Source: CAD feature listing. Evaluate the final solid. Frame: model axes, mm. A direction names the side the tool comes from. Round coordinates to 2 decimals unless told otherwise and drop trailing zeros. Order: outer loops, then holes, each group sorted by start corner. A loop starts at its lowest first (then second) coordinate and runs counter-clockwise, first axis right, second up. Notation, with made-up numbers: M 47,16.5 L 87,16.5 A22 ccw 87,39.5 Z; hole C -15,80 d9. An arc over 180 degrees is marked long. Use one line per item in the form item = value. Start each with the question number.
Q1. Section C-C (x = 38.5). Return the cut outline in (y, z), plus the area to 3 significant figures.
Q2. Material intervals for probe 1 along Y at (x, z) = (53.5, 0); probe 2 along X at (y, z) = (34, 315); probe 3 along X at (y, z) = (-11, 305.5), sorted ascending.
Q3. Section D-D (y = 18.5). Return the cut outline in (x, z).
Q4. Contact query for flat-ended pins moving along their axis: pin 1 (18 mm diameter, centred on y = 3.5, z = 301, fed in from +X); pin 2 (3.5 mm diameter, centred on y = -1, z = -1.5, fed in from -X); pin 3 (12 mm diameter, centred on x = 21, z = 171.5, fed in from +Y). Output: stop coordinate, or through.
Q5. Pull-direction query (Z, two-part tool) for faces 6 (the flat face through (30, -30, 157)), 7 (the cylindrical face through (-4.93, -3.651, 305.217)), 8 (the flat face through (0, -8, 311)); classes: pulls with the +Z half, pulls with the -Z half, needs draft (parallel to the pull), parting line crosses it, or undercut.
Q6. Section B-B (y = 0). Return the cut outline in (x, z).
Q7. Reachability of faces 1 (the flat face through (60, 30, -6)), 2 (the cylindrical face through (5, 0, -6)), 3 (the flat face through (50, 0, 0)), 4 (the flat face through (0, 1, -8)), 5 (the flat face through (30, 30, 157)) from +Z, -Z, +X, -X, +Y, -Y: full face, straight path, thin tool, end or side. Return the list, or none.
Q8. Section A-A (z = 0). Return the cut outline in (x, y).
from build123d import *

# Parameters (mm, degrees)
SKETCH1_R             = 40
BOSS_EXTRUDE1_DEPTH   = 60
BOSS_EXTRUDE1_2_DEPTH = 60
BOSS_EXTRUDE2_START   = -121.840385
SKETCH5_W             = 40
SKETCH5_H             = 60
BOSS_EXTRUDE2_DEPTH   = 257.063378
SKETCH7_R             = 6
CUT_EXTRUDE5_DEPTH    = 10
SKETCH8_R             = 6
BOSS_EXTRUDE3_DEPTH   = 10
SKETCH2_R             = 30
CUT_EXTRUDE6_DEPTH    = 10


with BuildPart() as part:
    # Sketch1 → Boss-Extrude1 (new body)
    with BuildSketch(Plane(origin=(0, 0, 0), x_dir=(0, 0, -1), z_dir=(1, 0, 0))):
        Circle(SKETCH1_R)
    extrude(amount=BOSS_EXTRUDE1_DEPTH)



with BuildPart() as body_2:
    # Sketch1 → Boss-Extrude1 2 (new body)
    with BuildSketch(Plane(origin=(0, 0, 0), x_dir=(0, 0, -1), z_dir=(1, 0, 0))):
        with Locations((-309.978404015, 0)):
            Circle(SKETCH1_R)
    extrude(amount=BOSS_EXTRUDE1_2_DEPTH)


with BuildPart() as part_1:
    add(part.part)

    add(body_2.part)  # Boss-Extrude2 merges body 2
    # Sketch5 → Boss-Extrude2 (add)
    with BuildSketch(Plane(origin=(0, 0, 161.680506403), x_dir=(-1, 0, 0), z_dir=(0, 0, -1)).offset(BOSS_EXTRUDE2_START)):
        with Locations((-30, 0)):
            Rectangle(SKETCH5_W, SKETCH5_H)
    extrude(amount=BOSS_EXTRUDE2_DEPTH)

    # Sketch7 → Cut-Extrude5 (cut)
    with BuildSketch(Plane.ZY):
        Circle(SKETCH7_R)
    extrude(amount=-CUT_EXTRUDE5_DEPTH, mode=Mode.SUBTRACT)

    # Sketch8 → Boss-Extrude3 (add)
    with BuildSketch(Plane.ZY):
        with Locations((309.978404015, 0)):
            Circle(SKETCH8_R)
    extrude(amount=BOSS_EXTRUDE3_DEPTH)

    # Sketch2 → Cut-Extrude6 (cut)
    with BuildSketch(Plane(origin=(60, 0, 0), x_dir=(0, 0, -1), z_dir=(1, 0, 0))):
        Circle(SKETCH2_R)
        with Locations((-309.978404015, 0)):
            Circle(SKETCH2_R)
    extrude(amount=-CUT_EXTRUDE6_DEPTH, mode=Mode.SUBTRACT)


solid = part_1.part
Results list:
q1.outline = M -30,26.46 A40 ccw long 30,26.46 L 30,283.52 A40 ccw long -30,283.52 Z
q1.area = 24,400 mm2
q2.probe_1 = -40 to -30, 30 to 40
q2.probe_2 = 0 to 60
q2.probe_3 = 0 to 50
q3.outline = M 0,-35.46 L 60,-35.46 L 60,-23.62 L 50,-23.62 L 50,23.62 L 60,23.62 L 60,35.46 L 50,35.46 L 50,274.51 L 60,274.51 L 60,286.36 L 50,286.36 L 50,333.6 L 60,333.6 L 60,345.44 L 0,345.44 L 0,274.51 L 10,274.51 L 10,35.46 L 0,35.46 Z
q4.pin_1 = 50
q4.pin_2 = 10
q4.pin_3 = 30
q5.face_6 = undercut
q5.face_7 = parting line crosses it
q5.face_8 = needs draft
q6.outline = M -10,303.98 L 0,303.98 L 0,269.98 L 10,269.98 L 10,40 L 0,40 L 0,6 L 10,6 L 10,-6 L 0,-6 L 0,-40 L 60,-40 L 60,-30 L 50,-30 L 50,30 L 60,30 L 60,40 L 50,40 L 50,269.98 L 60,269.98 L 60,279.98 L 50,279.98 L 50,339.98 L 60,339.98 L 60,349.98 L 0,349.98 L 0,315.98 L -10,315.98 Z
q7.face_1 = +Z, -Z, +X, +Y, -Y
q7.face_2 = -X
q7.face_3 = +X
q7.face_4 = -Z, -X, +Y, -Y
q7.face_5 = +X, -X, +Y
q8.outline = M 0,-40 L 60,-40 L 60,-30 L 50,-30 L 50,30 L 60,30 L 60,40 L 0,40 L 0,6 L 10,6 L 10,-6 L 0,-6 Z
